Autodesk Inventor part; units mm, degrees
ref_plane "YZ Plane" through (0, 0, 0) normal (1, 0, 0) x (0, 1, 0)
ref_plane "XZ Plane" through (0, 0, 0) normal (0, 1, 0) x (-1, 0, 0)
ref_plane "XY Plane" through (0, 0, 0) normal (0, 0, 1) x (1, 0, 0)
sketch "Sketch1" plane through (0, 0, 0) normal (0, 1, 0) x (-1, 0, 0)
  line L0 (0, 0) -> (0, -225.149) construction
  line L1 (-5, 0) -> (-5, -225.149)
  line L2 (5, -225.149) -> (5, 0)
  arc A0 (5, 0) -> (-5, 0) centre (0, 0) ccw
  arc A1 (-5, -225.149) -> (5, -225.149) centre (0, -225.149) ccw
  circle A2 centre (0, 0) radius 1.5
  circle A3 centre (0, -225.149) radius 1.5
  point P0 (0, -112.5745)
  dimension "d0" = 225.149
  dimension "d1" = 10
  dimension "d2" = 3
  dimension "d3" = 3
extrude "Extrusion1" add sketch "Sketch1" along normal blind 8
sketch "Sketch2" plane through (0, 8, 0) normal (0, 1, 0) x (1, 0, 0)
  arc A0 (5, 225.149) -> (-5, 225.149) centre (0, 225.149) ccw
  line L0 (-5, 225.149) -> (-5, 0)
  arc A1 (-5, 0) -> (5, 0) centre (0, 0) ccw
  line L1 (5, 0) -> (5, 225.149)
  circle A2 centre (0, 225.149) radius 1.5
  circle A3 centre (0, 0) radius 1.5
  circle A4 centre (0, 225.149) radius 5
  point P0 (-5, 225.149)
  point P1 (5, 225.149)
  dimension "d12" = 10
extrude "Extrusion2" add sketch "Sketch2" along normal blind 8 contours A4 A0
sketch "Sketch3" plane through (0, 0, 0) normal (0, -1, 0) x (1, 0, 0)
  arc A0 (-5, -225.149) -> (5, -225.149) centre (0, -225.149) ccw
  line L0 (5, 0) -> (5, -225.149)
  arc A1 (5, 0) -> (-5, 0) centre (0, 0) ccw
  line L1 (-5, -225.149) -> (-5, 0)
  circle A2 centre (0, -225.149) radius 1.5
  circle A3 centre (0, 0) radius 1.5
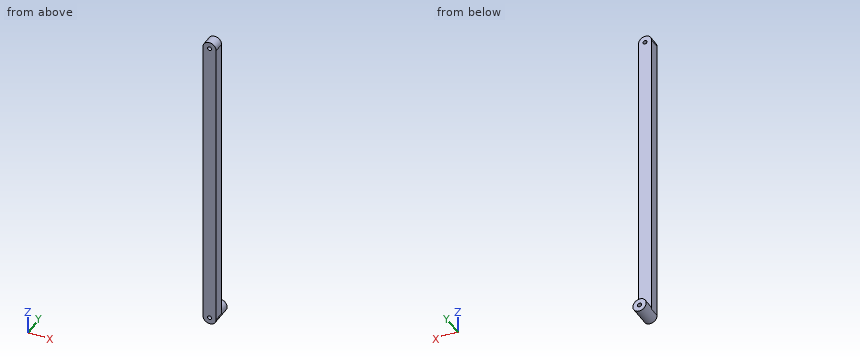
Read the model definition and answer for the solid it produces. Units are mm, in the model's axes. Give positions to 0.01 mm unless a question says otherwise; leave off trailing zeros. Loops run counter-clockwise (first coordinate to the right, second up) from the corner with the lowest first, then second, coordinate; pieces in that order, holes last.
Item 1: Each of these flat-tipped pins is pushed along its axis until it touches: pin 1 Ø5 at (x, y) = (1.5, 13.5) entering from +Z; pin 2 Ø1.5 at (x, y) = (1.5, 7.5) entering from +Z; pin 3 Ø1.8 at (x, z) = (0, 0) entering from -Y. Where does it stop, or does it pass through?
Item 2: The part is cut by section B-B (z = -131). Write down the section's boundary in (x, y).
Item 3: Find the intervals of material crossed by line 1 along Z through (x, y) = (0, 4); line 2 along Z through (x, y) = (0.25, 1.25); line 3 along Y through (x, z) = (-3.5, -199), in increasing order.
Taken from the geometry:
1. pin 1: stops at z = -220.15
1. pin 2: stops at z = 4.94
1. pin 3: passes through
2. outline: (-5, 0) - (5, 0) - (5, 8) - (-5, 8) - close
3. line 1: z = -230.15 to -226.65, -223.65 to -1.5, 1.5 to 5
3. line 2: z = -230.14 to -226.63, -223.67 to -1.48, 1.48 to 4.99
3. line 3: y = 0 to 8
